```python
from build123d import *

# Parameters (mm, degrees)
SKETCH1_R           = 2.5
SKETCH1_R_2         = 1.016
SKETCH1_R_3         = 0.080960088
BOSS_EXTRUDE1_DEPTH = 1.55
CUT_EXTRUDE1_DEPTH  = 2.55
CUT_EXTRUDE2_DEPTH  = 2.55


with BuildPart() as part:
    # Sketch1 → Boss-Extrude1 (new body)
    with BuildSketch(Plane(origin=(0, 0, 0), x_dir=(1, 0, 0), z_dir=(0, 1, 0))):
        with BuildLine():
            Line((-23.244816627, 44.45), (23.244816627, 44.45))
            ThreePointArc((23.244816627, 44.45), (24.583514169, 44.270437622), (25.827574029, 43.744444444))
            ThreePointArc((25.827574029, 43.744444444), (35.740062311, 36.101079569), (43.482663438, 26.265909091))
            ThreePointArc((43.482663438, 26.265909091), (45.334600658, 24.468164919), (47.830929781, 23.8125))
            Line((47.830929781, 23.8125), (71.516875, 23.8125))
            Line((71.516875, 23.8125), (76.596875, 18.7325))
            Line((76.596875, 18.7325), (76.596875, -18.7325))
            Line((76.596875, -18.7325), (71.516875, -23.8125))
            Line((71.516875, -23.8125), (47.830929781, -23.8125))
            ThreePointArc((47.830929781, -23.8125), (45.334600658, -24.468164919), (43.482663438, -26.265909091))
            ThreePointArc((43.482663438, -26.265909091), (35.740062311, -36.101079569), (25.827574029, -43.744444444))
            ThreePointArc((25.827574029, -43.744444444), (24.583514169, -44.270437622), (23.244816627, -44.45))
            Line((23.244816627, -44.45), (-23.244816627, -44.45))
            ThreePointArc((-23.244816627, -44.45), (-24.583514169, -44.270437622), (-25.827574029, -43.744444444))
            ThreePointArc((-25.827574029, -43.744444444), (-35.740062311, -36.101079569), (-43.482663438, -26.265909091))
            ThreePointArc((-43.482663438, -26.265909091), (-45.334600658, -24.468164919), (-47.830929781, -23.8125))
            Line((-47.830929781, -23.8125), (-71.516875, -23.8125))
            Line((-71.516875, -23.8125), (-76.596875, -18.7325))
            Line((-76.596875, -18.7325), (-76.596875, 18.7325))
            Line((-76.596875, 18.7325), (-71.516875, 23.8125))
            Line((-71.516875, 23.8125), (-47.830929781, 23.8125))
            ThreePointArc((-47.830929781, 23.8125), (-45.334600658, 24.468164919), (-43.482663438, 26.265909091))
            ThreePointArc((-43.482663438, 26.265909091), (-35.740062311, 36.101079569), (-25.827574029, 43.744444444))
            ThreePointArc((-25.827574029, 43.744444444), (-24.583514169, 44.270437622), (-23.244816627, 44.45))
        make_face()
        Circle(SKETCH1_R, mode=Mode.SUBTRACT)
        with Locations((36.819050096, 28.19800422)):
            Circle(SKETCH1_R_2, mode=Mode.SUBTRACT)
        with Locations((28.19800422, 36.819050096)):
            Circle(SKETCH1_R_2, mode=Mode.SUBTRACT)
        with Locations((26.671582547, 26.671582547)):
            Circle(SKETCH1_R_3, mode=Mode.SUBTRACT)
        with Locations((26.671582547, -26.671582547)):
            Circle(SKETCH1_R_3, mode=Mode.SUBTRACT)
        with Locations((36.819050096, -28.19800422)):
            Circle(SKETCH1_R_2, mode=Mode.SUBTRACT)
        with Locations((28.19800422, -36.819050096)):
            Circle(SKETCH1_R_2, mode=Mode.SUBTRACT)
        with Locations((-26.671582547, -26.671582547)):
            Circle(SKETCH1_R_3, mode=Mode.SUBTRACT)
        with Locations((-28.19800422, -36.819050096)):
            Circle(SKETCH1_R_2, mode=Mode.SUBTRACT)
        with Locations((-36.819050096, -28.19800422)):
            Circle(SKETCH1_R_2, mode=Mode.SUBTRACT)
        with Locations((-26.671582547, 26.671582547)):
            Circle(SKETCH1_R_3, mode=Mode.SUBTRACT)
        with Locations((-36.819050096, 28.19800422)):
            Circle(SKETCH1_R_2, mode=Mode.SUBTRACT)
        with Locations((-28.19800422, 36.819050096)):
            Circle(SKETCH1_R_2, mode=Mode.SUBTRACT)
    extrude(amount=BOSS_EXTRUDE1_DEPTH)

    # Sketch2 → Cut-Extrude1 (cut, through all)
    with BuildSketch(Plane(origin=(0, 1.55, 0), x_dir=(1, 0, 0), z_dir=(0, 1, 0))):
        with BuildLine():
            Line((48, 15), (68, 15))
            ThreePointArc((68, 15), (70, 13), (68, 11))
            Line((68, 11), (48, 11))
            ThreePointArc((48, 11), (46, 13), (48, 15))
        make_face()
        with BuildLine():
            Line((48, -15), (68, -15))
            ThreePointArc((68, -15), (70, -13), (68, -11))
            Line((68, -11), (48, -11))
            ThreePointArc((48, -11), (46, -13), (48, -15))
        make_face()
        with BuildLine():
            Line((-48, 15), (-68, 15))
            ThreePointArc((-68, 15), (-70, 13), (-68, 11))
            Line((-68, 11), (-48, 11))
            ThreePointArc((-48, 11), (-46, 13), (-48, 15))
        make_face()
        with BuildLine():
            Line((-48, -15), (-68, -15))
            ThreePointArc((-68, -15), (-70, -13), (-68, -11))
            Line((-68, -11), (-48, -11))
            ThreePointArc((-48, -11), (-46, -13), (-48, -15))
        make_face()
    extrude(amount=-CUT_EXTRUDE1_DEPTH, mode=Mode.SUBTRACT)

    # Sketch3 → Cut-Extrude2 (cut, through all)
    with BuildSketch(Plane(origin=(0, 1.55, 0), x_dir=(1, 0, 0), z_dir=(0, 1, 0))):
        with BuildLine():
            Line((-11, 33), (11, 33))
            ThreePointArc((11, 33), (13.121320344, 32.121320344), (14, 30))
            Line((14, 30), (14, 26))
            ThreePointArc((14, 26), (13.121320344, 23.878679656), (11, 23))
            Line((11, 23), (-11, 23))
            ThreePointArc((-11, 23), (-13.121320344, 23.878679656), (-14, 26))
            Line((-14, 26), (-14, 30))
            ThreePointArc((-14, 30), (-13.121320344, 32.121320344), (-11, 33))
        make_face()
        with BuildLine():
            Line((14, -30), (14, -26))
            ThreePointArc((14, -26), (13.121320344, -23.878679656), (11, -23))
            Line((11, -23), (-11, -23))
            ThreePointArc((-11, -23), (-13.121320344, -23.878679656), (-14, -26))
            Line((-14, -26), (-14, -30))
            ThreePointArc((-14, -30), (-13.121320344, -32.121320344), (-11, -33))
            Line((-11, -33), (11, -33))
            ThreePointArc((11, -33), (13.121320344, -32.121320344), (14, -30))
        make_face()
        with BuildLine():
            Line((31, 14), (35, 14))
            ThreePointArc((35, 14), (37.121320344, 13.121320344), (38, 11))
            Line((38, 11), (38, -11))
            ThreePointArc((38, -11), (37.121320344, -13.121320344), (35, -14))
            Line((35, -14), (31, -14))
            ThreePointArc((31, -14), (28.878679656, -13.121320344), (28, -11))
            Line((28, -11), (28, 11))
            ThreePointArc((28, 11), (28.878679656, 13.121320344), (31, 14))
        make_face()
        with BuildLine():
            Line((-38, 11), (-38, -11))
            ThreePointArc((-38, -11), (-37.121320344, -13.121320344), (-35, -14))
            Line((-35, -14), (-31, -14))
            ThreePointArc((-31, -14), (-28.878679656, -13.121320344), (-28, -11))
            Line((-28, -11), (-28, 11))
            ThreePointArc((-28, 11), (-28.878679656, 13.121320344), (-31, 14))
            Line((-31, 14), (-35, 14))
            ThreePointArc((-35, 14), (-37.121320344, 13.121320344), (-38, 11))
        make_face()
    extrude(amount=-CUT_EXTRUDE2_DEPTH, mode=Mode.SUBTRACT)


solid = part.part
```
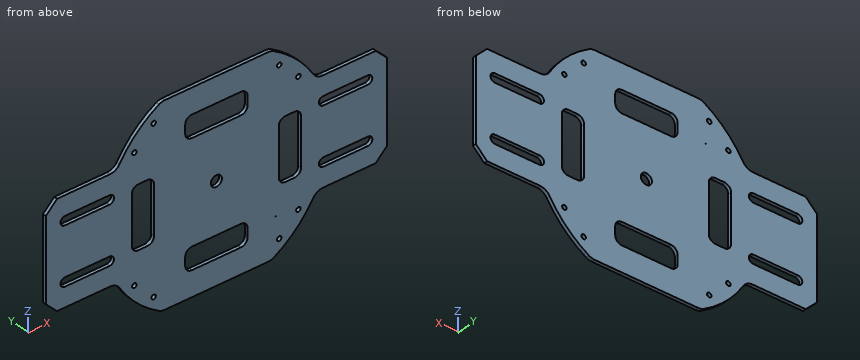
Here's how the part is built. I have some questions about the finished solid (model axes, mm). Give positions to 0.01 mm unless a question says otherwise; leave off trailing zeros. Order: outer loops, then holes, each group sorted by start corner. A loop starts at its lowest first (then second) coordinate and runs counter-clockwise, first axis right, second up. Notation, with made-up numbers: M 27.25,73 L 65.25,73 A21 cw 65.25,104 Z; hole C 66,-15.5 d7. An arc over 180 degrees is marked long. Use a Markdown table: item, result. Add a question column.
1. I need wall thicknesses on probe 1 along Z at (x, y) = (48, 0.1); probe 2 along X at (y, z) = (0.75, 0); probe 3 along Z at (x, y) = (0, 1.1). Which ranges of each line are inside material? Lowest first, please. Write a range as from..to.
2. Suppose I cut it at C-C (x = -56.5). List the corners of the cut face in (y, z) for me, and give its area (3 significant figures).
3. For pin 1 Ø0.8 at (x, y) = (-58.5, 0.5) entering from -Z, with a flat end and sliding along its axis, tell me the tip position at first contact or that it passes through.
4. Suppose I cut it at D-D (y = 1). Give the number of separate pieces and of enclosed holes in the cut face, and give its area (3 significant figures).
5. Suppose I cut it at B-B (x = 0). List the corners of the cut face in (y, z) for me.
6. Suppose I cut it at A-A (z = 0). List the corners of the cut face in (x, y) for me.
Results list:
| question | item | result |
|---|---|---|
| 1 | probe 1 | z = -23.81..-15, -11..11, 15..23.81 |
| 1 | probe 2 | x = -76.6..-38, -28..-2.5, 2.5..28, 38..76.6 |
| 1 | probe 3 | z = -44.45..-33, -23..-2.5, 2.5..23, 33..44.45 |
| 2 | outline | M 0,-23.81 L 1.55,-23.81 L 1.55,-15 L 0,-15 Z; M 0,-11 L 1.55,-11 L 1.55,11 L 0,11 Z; M 0,15 L 1.55,15 L 1.55,23.81 L 0,23.81 Z |
| 2 | area | 61.4 mm² |
| 3 | pin 1 | stops at z = -23.81 |
| 4 | separate pieces | 1 |
| 4 | enclosed holes | 21 |
| 4 | area | 8,770 mm² |
| 5 | outline | M 0,-44.45 L 1.55,-44.45 L 1.55,-33 L 0,-33 Z; M 0,-23 L 1.55,-23 L 1.55,-2.5 L 0,-2.5 Z; M 0,2.5 L 1.55,2.5 L 1.55,23 L 0,23 Z; M 0,33 L 1.55,33 L 1.55,44.45 L 0,44.45 Z |
| 6 | outline | M -76.6,0 L -38,0 L -38,1.55 L -76.6,1.55 Z; M -28,0 L -2.5,0 L -2.5,1.55 L -28,1.55 Z; M 2.5,0 L 28,0 L 28,1.55 L 2.5,1.55 Z; M 38,0 L 76.6,0 L 76.6,1.55 L 38,1.55 Z |
